CAD build for the part. Positions are in the model's coordinates, mm. Round coordinates to 2 decimals unless told otherwise and drop trailing zeros. Order: outer loops, then holes, each group sorted by start corner. A loop starts at its lowest first (then second) coordinate and runs counter-clockwise, first axis right, second up. Notation, with made-up numbers: (66.25, -24) - (75.25, -24) arc R21 cw to (75.25, -18) - close; hole circle Ø4 at (47.5, 77.25). An arc over 180 degrees is marked (long way). Write item = value, one per line.
Autodesk Inventor part; units mm, degrees
sketch "Sketch1" plane through (0, 0, 0) normal (0, 0, 1) x (1, 0, 0)
  line L0 (0, 2.8582) -> (0, -2.8582) construction
  line L1 (-5.7775, 0) -> (5.7775, 0) construction
  circle A0 centre (0, 0) radius 25.629
  circle A1 centre (0, 0) radius 4
  line L2 (0, 4) -> (0, 7)
  line L3 (0, 7) -> (0, 21)
  line L4 (0, 21) -> (5, 21)
  line L5 (5, 21) -> (8, 21)
  line L6 (8, 21) -> (0, 7)
  line L7 (0, 21) -> (-8, 21)
  line L8 (-8, 21) -> (0, 7)
  line L9 (0, -4) -> (0, -7)
  line L10 (0, -7) -> (0, -21)
  line L11 (0, -21) -> (8, -21)
  line L12 (8, -21) -> (0, -7)
  line L13 (0, -21) -> (-8, -21)
  line L14 (-8, -21) -> (0, -7)
  line L15 (0, 0) -> (2.5981, 1.5)
  line L16 (0, 0) -> (3, 0) construction
  line L17 (2.5981, 1.5) -> (3.4641, 2)
  line L18 (3.4641, 2) -> (6.0622, 3.5)
  line L19 (6.0622, 3.5) -> (18.1865, 10.5)
  line L20 (18.1865, 10.5) -> (14.1865, 17.4282)
  line L21 (14.1865, 17.4282) -> (6.0622, 3.5)
  line L22 (18.1865, 10.5) -> (22.1865, 3.5718)
  line L23 (22.1865, 3.5718) -> (6.0622, 3.5)
  line L24 (0, 0) -> (8, 0) construction
  line L25 (0, 0) -> (3.4641, -2)
  line L26 (0, 0) -> (4, 0) construction
  line L27 (3.4641, -2) -> (6.0622, -3.5)
  line L28 (6.0622, -3.5) -> (18.1865, -10.5)
  line L29 (18.1865, -10.5) -> (14.1865, -17.4282)
  line L30 (14.1865, -17.4282) -> (6.0934, -3.518)
  line L31 (18.1865, -10.5) -> (22.0919, -3.518)
  line L32 (22.0919, -3.518) -> (6.0934, -3.518)
  line L33 (0, 0) -> (-2.5981, 1.5)
  line L34 (0, 0) -> (3, 0) construction
  line L35 (-2.5981, 1.5) -> (-3.4641, 2)
  line L36 (-3.4641, 2) -> (-6.0622, 3.5)
  line L37 (-6.0622, 3.5) -> (-18.1865, 10.5)
  line L38 (-18.1865, 10.5) -> (-14.1865, 17.4282)
  line L39 (-14.1865, 17.4282) -> (-6.0622, 3.5)
  line L40 (-18.1865, 10.5) -> (-22.1865, 3.5718)
  line L41 (-22.1865, 3.5718) -> (-6.0622, 3.5)
  line L42 (0, 0) -> (-6.0622, -3.5)
  line L43 (0, 0) -> (7, 0) construction
  line L44 (-6.0622, -3.5) -> (-18.1865, -10.5)
  line L45 (-18.1865, -10.5) -> (-14.1865, -17.4282)
  line L46 (-14.1865, -17.4282) -> (-6.0622, -3.5)
  line L47 (-18.1865, -10.5) -> (-22.1865, -3.5718)
  line L48 (-22.1865, -3.5718) -> (-6.0622, -3.5)
  dimension "d0" = 51.258
  dimension "d1" = 8
  dimension "d2" = 3
  dimension "d3" = 14
  dimension "d4" = 5
  dimension "d5" = 3
  dimension "d6" = 8
  dimension "d7" = 3
  dimension "d8" = 14
  dimension "d9" = 8
  dimension "d10" = 8
  dimension "d11" = 3
  dimension "d12" = 30
  dimension "d13" = 3
  dimension "d14" = 14
  dimension "d15" = 8
  dimension "d16" = 8
  dimension "d19" = 4
  dimension "d20" = 30
  dimension "d21" = 3
  dimension "d22" = 14
  dimension "d23" = 8
  dimension "d24" = 8
  dimension "d25" = 3
  dimension "d26" = 150
  dimension "d27" = 1
  dimension "d28" = 180
  dimension "d29" = 3
  dimension "d30" = 180
  dimension "d31" = 180
  dimension "d32" = 8
  dimension "d33" = 8
  dimension "d34" = 7
  dimension "d35" = 150
  dimension "d36" = 14
  dimension "d37" = 180
  dimension "d38" = 8
  dimension "d39" = 8
extrude "Extrusion1" add sketch "Sketch1" along normal blind 2
fillet "Fillet1" radius 2 18 edges at (14.1865, 17.4282, 1) (22.1865, 3.5718, 1) (6.0622, 3.5, 1) (22.0919, -3.518, 1) (14.1865, -17.4282, 1) (6.0934, -3.518, 1) (0, 7, 1) (-8, 21, 1) (8, 21, 1) (-6.0622, 3.5, 1) (-22.1865, 3.5718, 1) (-14.1865, 17.4282, 1) (-6.0622, -3.5, 1) (-14.1865, -17.4282, 1) (-22.1865, -3.5718, 1) (-8, -21, 1) (0, -7, 1) (8, -21, 1)
sketch "Sketch2" plane through (0, 0, 2) normal (0, 0, 1) x (1, 0, 0)
  circle A0 centre (0, 0) radius 3.05
  circle A1 centre (0, 0) radius 5
  dimension "d43" = 6.1
  dimension "d49" = 10
extrude "Extrusion2" add sketch "Sketch2" against normal blind 2
chamfer "Chamfer1" distance 1 angle 45 1 edges at (-25.629, 0, 2)
properties part number "Wiel hout" material "S235"
(1) Band-saw the part on C-C on z = 1.4. Count the separate pieces of the cut face and the enclosed holes in it, plus the area to 3 significant figures.
Solved:
separate_pieces = 1
enclosed_holes = 7
area = 1,350 mm²
(2) Band-saw the part on A-A on y = 0. List the corners of the cut face in (x, z).
Solved:
outline = (-25.63, 0) - (-3.05, 0) - (-3.05, 2) - (-24.63, 2) - (-25.63, 1) - close; (3.05, 0) - (25.63, 0) - (25.63, 1) - (24.63, 2) - (3.05, 2) - close
(3) Probe line 1 along Y through (x, z) = (0, 0.7); line 2 along Y through (x, z) = (13, 1.9); line 3 along Y through (x, z) = (-0.5, 1.55). List the from-to ranges inside material, lowest first.
Solved:
line_1 = -25.63 to -21, -9.03 to -3.05, 3.05 to 9.03, 21 to 25.63
line_2 = -21.04 to -15.05, -3.52 to 3.53, 15.06 to 21.04
line_3 = -25.07 to -21, -9.09 to -3.01, 3.01 to 9.09, 21 to 25.07
(4) Pull direction Y, two halves, no side cores. Call faces 1 (the cylindrical face through (-7.807, -4.541, 1.014)), 2 (the cylindrical face through (14.211, 15.443, 1.014)), 3 (the cylindrical face through (-20.34, 15.59, 0.49)): released by +Y, released by -Y, zero draft, split by the parting line, or undercut.
Solved:
face_1 = undercut
face_2 = undercut
face_3 = split by the parting line
(5) Drop flat-ended pins along their axis: pin 1 (1 mm diameter, centred on x = 20, y = -6, fed in from +Z); pin 2 (8 mm diameter, centred on x = 13, y = -6.5, fed in from -Z); pin 3 (0.6 mm diameter, centred on x = 14, z = 1, fed in from -Y). Give the stop position or say it passes through.
Solved:
pin_1 = through
pin_2 = 0
pin_3 = -21.66
(6) Band-saw the part on B-B on x = 0. List the corners of the cut face in (y, z), plus the area to 3 significant figures.
Solved:
outline = (-25.63, 0) - (-21, 0) - (-21, 2) - (-24.63, 2) - (-25.63, 1) - close; (-9.03, 0) - (-3.05, 0) - (-3.05, 2) - (-9.03, 2) - close; (3.05, 0) - (9.03, 0) - (9.03, 2) - (3.05, 2) - close; (21, 0) - (25.63, 0) - (25.63, 1) - (24.63, 2) - (21, 2) - close
area = 41.4 mm²
